Input: part model. Units: mm. Frame: model coordinates. A direction names the side the tool comes from. Coordinates: 2 decimals unless noted, no trailing zeros. Order: outer loops, then holes, each group sorted by start corner. A loop starts at its lowest first (then second) coordinate and runs counter-clockwise, first axis right, second up. Notation, with made-up numbers: (50.5, 64.5) - (62.5, 64.5) arc R17 cw to (62.5, 82.5) - close; hole circle Ø8 at (60, 37.25). An arc over 180 degrees is marked (long way). One line per question, with ' | ' between items. Start each with the question number.
Autodesk Inventor part; units mm, degrees
ref_plane "YZ Plane" through (0, 0, 0) normal (1, 0, 0) x (0, 1, 0)
ref_plane "XZ Plane" through (0, 0, 0) normal (0, 1, 0) x (-1, 0, 0)
ref_plane "XY Plane" through (0, 0, 0) normal (0, 0, 1) x (1, 0, 0)
sketch "Sketch1" plane through (0, 0, 0) normal (0, 0, 1) x (1, 0, 0)
  circle A0 centre (0, 0) radius 7.5
  line L0 (-5.7735, 0) -> (-2.8868, 5)
  line L1 (-2.8868, 5) -> (2.8868, 5)
  line L2 (2.8868, 5) -> (5.7735, 0)
  line L3 (5.7735, 0) -> (2.8868, -5)
  line L4 (2.8868, -5) -> (-2.8868, -5)
  line L5 (-2.8868, -5) -> (-5.7735, 0)
  dimension "d0" = 15
  dimension "d1" = 10
extrude "Extrusion1" add sketch "Sketch1" along normal blind 9 contours A0 | L0 L1 L2 L3 L4 L5
sketch "Sketch4" plane through (0, 0, 9) normal (0, 0, 1) x (1, 0, 0)
  circle A0 centre (0, 0) radius 3
  dimension "d15" = 6
extrude "Extrusion4" cut sketch "Sketch4" against normal through all
sketch "Sketch5" plane through (0, 0, 9) normal (0, 0, 1) x (1, 0, 0)
  line L0 (-2.9156, -5.05) -> (-5.8312, 0)
  line L1 (-5.8312, 0) -> (-2.9156, 5.05)
  line L2 (-2.9156, 5.05) -> (2.9156, 5.05)
  line L3 (2.9156, 5.05) -> (5.8312, 0)
  line L4 (5.8312, 0) -> (2.9156, -5.05)
  line L5 (2.9156, -5.05) -> (-2.9156, -5.05)
  point P0 (0, 0)
  point P1 (0, 0)
  dimension "d18" = 10.1
extrude "Extrusion5" cut sketch "Sketch5" against normal blind 6
sketch "Sketch6" plane through (0, 0, 9) normal (0, 0, 1) x (1, 0, 0)
  point P0 (0, 0)
fillet "Fillet1" radius 2.1 6 edges at (5.8312, 0, 6) (2.9156, 5.05, 6) (-2.9156, 5.05, 6) (-5.8312, 0, 6) (-2.9156, -5.05, 6) (2.9156, -5.05, 6)
sketch "Sketch7" plane through (0, 0, 9) normal (0, 0, 1) x (1, 0, 0)
  arc A0 (-3.5218, -4) -> (-1.7032, -5.05) centre (-1.7032, -2.95) ccw
  arc A1 (-5.225, 1.05) -> (-5.225, -1.05) centre (-3.4064, 0) ccw
  arc A2 (-1.7032, 5.05) -> (-3.5218, 4) centre (-1.7032, 2.95) ccw
  arc A3 (3.5218, 4) -> (1.7032, 5.05) centre (1.7032, 2.95) ccw
  arc A4 (5.225, -1.05) -> (5.225, 1.05) centre (3.4064, 0) ccw
  arc A5 (1.7032, -5.05) -> (3.5218, -4) centre (1.7032, -2.95) ccw
  line L0 (-45.8, 0) -> (57.8, 0)
  circle A6 centre (-4.6441, 0) radius 1.2
  point P0 (0, 0)
  dimension "d22" = 2.4
extrude "Extrusion6" cut sketch "Sketch7" against normal up to surface (6 mm away)
pattern_circular "Circular Pattern1" count 6 over 360 about axis through (0, 0, 9) along (0, 0, -1) of "Extrusion6"
sketch "Sketch9" plane through (0, 0, 0) normal (0, 0, 1) x (1, 0, 0)
  line L0 (-10.5, 0) -> (10.5, 0)
  circle A0 centre (12.5, 0) radius 20 construction
  circle A1 centre (0, 0) radius 7.5
  line L1 (-7.5, -11.547) -> (-7.5, 11.547)
  line L2 (-7.5, 11.547) -> (12.5, 23.094)
  line L3 (12.5, 23.094) -> (32.5, 11.547)
  line L4 (32.5, 11.547) -> (32.5, -11.547)
  line L5 (32.5, -11.547) -> (12.5, -23.094)
  line L6 (12.5, -23.094) -> (-7.5, -11.547)
  point P0 (-7.5, 0)
  point P1 (-7.5, 0)
  dimension "d28" = 40
extrude "Extrusion7" add sketch "Sketch9" along normal up to surface (9 mm away)
sketch "Sketch10" plane through (10, 0, 9) normal (0, 0, 1) x (1, 0, 0)
  circle A0 centre (-6, -10) radius 2 construction
  point P0 (-10, 0)
  dimension "d31" = 4
  dimension "d32" = 4
  dimension "d33" = 10
fillet "Fillet2" radius 10 6 edges at (-7.5, -11.547, 4.5) (12.5, -23.094, 4.5) (32.5, -11.547, 4.5) (-7.5, 11.547, 4.5) (12.5, 23.094, 4.5) (32.5, 11.547, 4.5)
hole "Hole1" at (4, -10, 9) direction (0, 0, -1) diameter 5 end through all counterbore diameter 9 counterbore depth 0.8
sketch "Sketch13" plane through (0, 0, 0) normal (0, 0, -1) x (-1, 0, 0)
  circle A0 centre (-4, -10) radius 2.5
  line L0 (-8.05, -7.6617) -> (-4, -5.3235)
  line L1 (-4, -5.3235) -> (0.05, -7.6617)
  line L2 (0.05, -7.6617) -> (0.05, -12.3383)
  line L3 (0.05, -12.3383) -> (-4, -14.6765)
  line L4 (-4, -14.6765) -> (-8.05, -12.3383)
  line L5 (-8.05, -12.3383) -> (-8.05, -7.6617)
  line L6 (2.5, -14.4338) -> (-7.5, -20.2073)
  point P0 (0, 0)
  point P1 (-6.025, -13.5074)
  dimension "d44" = 8.1
extrude "Extrusion9" cut sketch "Sketch13" against normal blind 5.2
fillet "Fillet3" radius 2.1 6 edges at (4, -14.6765, 2.6) (-0.05, -12.3383, 2.6) (-0.05, -7.6617, 2.6) (4, -5.3235, 2.6) (8.05, -7.6617, 2.6) (8.05, -12.3383, 2.6)
sketch "Sketch15" plane through (0, 0, 0) normal (0, 0, -1) x (-1, 0, 0)
  arc A0 (-5.05, -14.0703) -> (-2.95, -14.0703) centre (-4, -12.2517) ccw
  line L0 (-4, -12.2517) -> (-4, -11.6129) construction
  circle A1 centre (-4, -13.3921) radius 1.25
  point P0 (0, 0)
  dimension "d48" = 2.5
extrude "Extrusion10" cut sketch "Sketch15" against normal up to surface (5.2 mm away)
pattern_circular "Circular Pattern2" count 6 over 360 about axis through (4, -10, -50.4819) along (0, 0, 1) of "Extrusion10"
sketch "Sketch16" plane through (0, 0, 9) normal (0, 0, 1) x (1, 0, 0)
  circle A0 centre (22.5, 0) radius 4
  line L0 (32.5, 5.7735) -> (32.5, -5.7735)
  point P0 (0, 0)
  dimension "d54" = 8
  dimension "d68" = 10
extrude "Extrusion11" cut sketch "Sketch16" against normal through all
sketch "Sketch17" plane through (0, 0, 0) normal (0, 0, -1) x (-1, 0, 0)
  circle A0 centre (-22.5, 0) radius 4
  line L0 (-29.05, -3.7816) -> (-29.05, 3.7816)
  line L1 (-29.05, 3.7816) -> (-22.5, 7.5633)
  line L2 (-22.5, 7.5633) -> (-15.95, 3.7816)
  line L3 (-15.95, 3.7816) -> (-15.95, -3.7816)
  line L4 (-15.95, -3.7816) -> (-22.5, -7.5633)
  line L5 (-22.5, -7.5633) -> (-29.05, -3.7816)
  line L6 (-32.5, -5.7735) -> (-32.5, 5.7735)
  point P0 (0, 0)
  dimension "d58" = 13.1
extrude "Extrusion12" cut sketch "Sketch17" against normal blind 5.5
fillet "Fillet4" radius 2.1 6 edges at (22.5, -7.5633, 2.75) (15.95, -3.7816, 2.75) (15.95, 3.7816, 2.75) (22.5, 7.5633, 2.75) (29.05, 3.7816, 2.75) (29.05, -3.7816, 2.75)
sketch "Sketch19" plane through (0, 0, 0) normal (0, 0, -1) x (-1, 0, 0)
  arc A0 (-23.55, -6.9571) -> (-21.45, -6.9571) centre (-22.5, -5.1384) ccw
  line L0 (-22.5, -5.1384) -> (-22.5, -8.2461) construction
  circle A1 centre (-22.5, -6.3761) radius 1.2
  arc A2 (-23.55, -6.9571) -> (-21.45, -6.9571) centre (-22.5, -5.1384) ccw
  line L1 (-21.45, -6.9571) -> (-22.5, -7.5633) construction
  line L2 (-23.55, -6.9571) -> (-22.5, -7.5633) construction
  line L3 (-23.55, -6.9571) -> (-28, -4.3879)
  point P0 (0, 0)
  dimension "d62" = 2.4
extrude "Extrusion13" cut sketch "Sketch19" against normal up to surface (5.5 mm away)
pattern_circular "Circular Pattern3" count 6 over 360 about axis through (22.5, 0, 9) along (0, 0, -1) of "Extrusion13"
sketch "Sketch20" plane through (0, 0, 5.5) normal (0, 0, -1) x (-1, 0, 0)
  circle A0 centre (-22.5, 0) radius 4
  circle A1 centre (-22.5, 0) radius 5.9
  point P0 (0, 0)
  dimension "d69" = 11.8
extrude "Extrusion14" cut sketch "Sketch20" against normal blind 0.65
sketch "Sketch21" plane through (0, 0, 9) normal (0, 0, 1) x (1, 0, 0)
  point P0 (0, 0)
sketch "Sketch22" plane through (0, 0, 9) normal (0, 0, 1) x (1, 0, 0)
  line L0 (54.5318, 10) -> (-19.1234, 10) construction
  arc A0 (32.5, 5.7735) -> (27.5, 14.4338) centre (22.5, 5.7735) ccw
  line L1 (-7.5, -5.7735) -> (-7.5, 5.7735)
  line L2 (15, 10) -> (10, 10) construction
  line L3 (15, 13) -> (10, 13)
  line L4 (10, 7) -> (15, 7)
  arc A1 (15, 7) -> (15, 13) centre (15, 10) ccw
  arc A2 (10, 13) -> (10, 7) centre (10, 10) ccw
  line L5 (12.5, 32) -> (12.5, -41) construction
  point P0 (0, 0)
  point P1 (12.5, 10)
  dimension "d72" = 40
  dimension "d74" = 6
  dimension "d75" = 5
  dimension "d76" = 10
  dimension "d79" = 20
extrude "Extrusion15" cut sketch "Sketch22" against normal blind 10
sketch "Sketch23" plane through (0, 0, 9) normal (0, 0, 1) x (1, 0, 0)
  arc A0 (15, 7) -> (15, 13) centre (15, 10) ccw
  circle A1 centre (22.5, 0) radius 4
  point P0 (0, 0)
sketch "Sketch24" plane through (0, 0, 0) normal (0, 0, -1) x (-1, 0, 0)
  arc A0 (7.5, 5.7735) -> (2.5, 14.4338) centre (-2.5, 5.7735) ccw
  line L0 (7.5, 5.7735) -> (7.5, 22) construction
  line L1 (-10, 7) -> (31, 7) construction
  point P0 (0, 0)
  point P1 (7.5, 7)
sketch "Sketch25" plane through (0, 0, 9) normal (0, 0, 1) x (1, 0, 0)
  arc A0 (-2.5, 14.4338) -> (-7.5, 5.7735) centre (2.5, 5.7735) ccw
  point P0 (0, 0)
  point P1 (-7.5, 7)
sketch "Sketch26" plane through (0, 0, 0) normal (0, 0, -1) x (-1, 0, 0)
  circle A0 centre (-4, -10) radius 2.5
  circle A1 centre (-22.5, 0) radius 4
  circle A2 centre (0, 0) radius 3
sketch "Sketch27" plane through (0, 0, 0) normal (0, 0, -1) x (-1, 0, 0)
  line L0 (-17, -4.3879) -> (-21.45, -6.9571)
  arc A0 (-23.55, -6.9571) -> (-21.45, -6.9571) centre (-22.5, -6.3761) ccw
  line L1 (-23.55, -6.9571) -> (-28, -4.3879)
  arc A1 (-29.05, -2.5692) -> (-28, -4.3879) centre (-28.0219, -3.1881) ccw
  line L2 (-29.05, -2.5692) -> (-29.05, 2.5692)
  arc A2 (-28, 4.3879) -> (-29.05, 2.5692) centre (-28.0219, 3.1881) ccw
  line L3 (-28, 4.3879) -> (-23.55, 6.9571)
  arc A3 (-21.45, 6.9571) -> (-23.55, 6.9571) centre (-22.5, 6.3761) ccw
  line L4 (-21.45, 6.9571) -> (-17, 4.3879)
  arc A4 (-15.95, 2.5692) -> (-17, 4.3879) centre (-16.9781, 3.1881) ccw
  line L5 (-15.95, 2.5692) -> (-15.95, -2.5692)
  arc A5 (-17, -4.3879) -> (-15.95, -2.5692) centre (-16.9781, -3.1881) ccw
  line L6 (-1, -12.9445) -> (-2.95, -14.0703)
  arc A6 (-5.05, -14.0703) -> (-2.95, -14.0703) centre (-4, -13.3921) ccw
  line L7 (-5.05, -14.0703) -> (-7, -12.9445)
  arc A7 (-8.05, -11.1258) -> (-7, -12.9445) centre (-6.9376, -11.696) ccw
  line L8 (-8.05, -11.1258) -> (-8.05, -8.8742)
  arc A8 (-7, -7.0555) -> (-8.05, -8.8742) centre (-6.9376, -8.304) ccw
  line L9 (-7, -7.0555) -> (-5.05, -5.9297)
  arc A9 (-2.95, -5.9297) -> (-5.05, -5.9297) centre (-4, -6.6079) ccw
  line L10 (-2.95, -5.9297) -> (-1, -7.0555)
  arc A10 (0.05, -8.8742) -> (-1, -7.0555) centre (-1.0624, -8.304) ccw
  line L11 (0.05, -8.8742) -> (0.05, -11.1258)
  arc A11 (-1, -12.9445) -> (0.05, -11.1258) centre (-1.0624, -11.696) ccw
  point P0 (0, 0)
sketch "Sketch28" plane through (0, 0, 9) normal (0, 0, 1) x (1, 0, 0)
  line L0 (-16.3382, 0) -> (43, 0) construction
  line L1 (12.5, 25) -> (12.5, -25) construction
  line L2 (32.5, 5.7735) -> (32.5, -5.7735)
  line L3 (-7.5, -5.7735) -> (-7.5, 5.7735)
  arc A0 (7.5, -20.2073) -> (17.5, -20.2073) centre (12.5, -11.547) ccw
  arc A1 (17.5, 20.2073) -> (7.5, 20.2073) centre (12.5, 11.547) ccw
  point P0 (0, 0)
  point P1 (-10.25, 24)
  dimension "d80" = 40
  dimension "d81" = 20
  dimension "d82" = 23.094
  dimension "d83" = 11.547
  dimension "d84" = 22.75
  dimension "d85" = 24
equation "\"d79\" = 0.5 * d72"
equation "\"d81\" = 0.5 * d80"
equation "\"d83\" = 0.5 * d82"
properties part number "Bottom"
(1) Pin query (flat end, axial travel): pin 1 (0.7 mm diameter, centred on y = -9.5, z = 2.5, fed in from -X); pin 2 (8 mm diameter, centred on x = 4, y = -10, fed in from +Z); pin 3 (2.5 mm diameter, centred on y = -9.5, z = 3.5, fed in from +X). Return the tip coordinate at first contact, or that it passes through.
(2) Material intervals for line 1 along Y through (x, z) = (4, 8.7); line 2 along Y through (x, z) = (0, 1.35); line 3 along X through (y, z) = (2, 5), sorted ascending. Write a range as from..to.
(3) Draft query along X for faces 4 (the face through (12, 0, 9)), 5 (the face through (2.43, 17.28, 4.44)), 6 (the face through (25.81, 5.65, 2.71)). Return one class per face: +X half, -X half, draft (parallel to the pull), parting line (faces both ways), or undercut.
(4) Section C-C (y = 10). Output: boundary loops of the cut face in (x, z).
(5) Section D-D (z = 1.5). State how many separate pieces and enclosed holes the cut face has, then the cut area to 3 significant figures.
(6) Reachability of faces 1 (the face through (15.95, 0, 3)), 2 (the face through (6, -12, 8.2)), 3 (the face through (-3, 0, 2)) from +Z, -Z, +X, -X, +Y, -Y: full face, straight path, thin tool, end or side. Return the list, or none.
(7) Section B-B (x = 13). Output: boundary loops of the cut face in (y, z), then the cut area to 3 significant figures.
(8) Section A-A (y = 0). Output: boundary loops of the cut face in (x, z), then the cut area to 3 significant figures.
Worked answers:
1) pin 1: stops at x = -6.91 | pin 2: stops at z = 8.2 | pin 3: stops at x = 32.19
2) line 1: y = -18.19..-14.5, -5.5..-3.17, 3.17..18.19 | line 2: y = -15.88..-12.35, -7.65..-3, 3..15.88 | line 3: x = -7.5..-4.68, 4.68..15.95, 29.05..32.5
3) face 4: draft | face 5: -X half | face 6: undercut
4) outline: (-6.56, 0) - (7, 0) - (7, 9) - (-6.56, 9) - close; (18, 0) - (31.56, 0) - (31.56, 9) - (18, 9) - close
5) separate pieces: 1 | enclosed holes: 4 | area: 1,060 mm²
6) face 1: -Z | face 2: +Z | face 3: +Z, -Z
7) outline: (-21.53, 0) - (7, 0) - (7, 9) - (-21.53, 9) - close; (13, 0) - (21.53, 0) - (21.53, 9) - (13, 9) - close | area: 334 mm²
8) outline: (-7.5, 0) - (-3, 0) - (-3, 3) - (-5.84, 3) - (-5.84, 9) - (-7.5, 9) - close; (3, 0) - (15.95, 0) - (15.95, 5.5) - (16.6, 5.5) - (16.6, 6.15) - (18.5, 6.15) - (18.5, 9) - (5.84, 9) - (5.84, 3) - (3, 3) - close; (26.5, 6.15) - (28.4, 6.15) - (28.4, 5.5) - (29.05, 5.5) - (29.05, 0) - (32.5, 0) - (32.5, 9) - (26.5, 9) - close | area: 169 mm²
